Can you work these out from the model? Positions are in its coordinate system, mm. Face numbers are marked on the shaded views. Round coordinates to 2 decimals unless told otherwise and drop trailing zeros. Loops run counter-clockwise (first coordinate to the right, second up) from the corner with the lowest first, then second, coordinate; pieces in that order, holes last. Notation, with made-up numbers: M 34,22 L 59,22 A25 ccw 59,54 Z; hole C -14.5,61 d1. An arc over 180 degrees is marked long. Return JSON: item names as keys, results as strings.
```python
from build123d import *

# Parameters (mm, degrees)
ESQUISSE1_R                = 20
ESQUISSE1_R_2              = 12
ESQUISSE1_R_3              = 1.15
BOSS_EXTRU_1_DEPTH         = 4
PER_AGEAVANC_1_OUTLINE_R   = 2.2
PER_AGEAVANC_1_OUTLINE_R_2 = 1.15
PER_AGEAVANC_1_DEPTH       = 2
BOSS_EXTRU_2_START         = -4
ESQUISSE3_R                = 13.45
ESQUISSE3_R_2              = 12
BOSS_EXTRU_2_DEPTH         = 2.3
CHANFREIN1_SIZE            = 0.5
CHANFREIN2_SIZE            = 1


# Read off the part's stored shape, not the designer's step: PerçageAvancé1
with BuildPart() as part:
    # Esquisse1 → Boss.-Extru.1 (new body)
    with BuildSketch(Plane(origin=(0, 0, 0), x_dir=(1, 0, 0), z_dir=(0, 1, 0))):
        with Locations(Location((0, 0, 0), (0, 0, 270))):
            Circle(ESQUISSE1_R)
        with Locations(Location((0, 0, 0), (0, 0, 270))):
            Circle(ESQUISSE1_R_2, mode=Mode.SUBTRACT)
        with Locations(Location((-14.289419162, -8.25, 0), (0, 0, 270))):
            Circle(ESQUISSE1_R_3, mode=Mode.SUBTRACT)
        with Locations(Location((14.289419162, -8.25, 0), (0, 0, 270))):
            Circle(ESQUISSE1_R_3, mode=Mode.SUBTRACT)
        with Locations(Location((0, 16.5, 0), (0, 0, 270))):
            Circle(ESQUISSE1_R_3, mode=Mode.SUBTRACT)
    extrude(amount=BOSS_EXTRU_1_DEPTH)

    # PerçageAvancé1 outline → PerçageAvancé1 (cut)
    # profile 1 of 3: a face of its own
    with BuildSketch(Plane(origin=(0, 0, 0), x_dir=(1, 0, 0), z_dir=(0, 1, 0))):
        with Locations((-14.289419162, -8.25)):
            Circle(PER_AGEAVANC_1_OUTLINE_R)
        with Locations((-14.289419162, -8.25)):
            Circle(PER_AGEAVANC_1_OUTLINE_R_2, mode=Mode.SUBTRACT)
    # profile 2 of 3: a face of its own
    with BuildSketch(Plane(origin=(0, 0, 0), x_dir=(1, 0, 0), z_dir=(0, 1, 0))):
        with Locations((14.289419162, -8.25)):
            Circle(PER_AGEAVANC_1_OUTLINE_R)
        with Locations((14.289419162, -8.25)):
            Circle(PER_AGEAVANC_1_OUTLINE_R_2, mode=Mode.SUBTRACT)
    # profile 3 of 3: a face of its own
    with BuildSketch(Plane(origin=(0, 0, 0), x_dir=(1, 0, 0), z_dir=(0, 1, 0))):
        with Locations((0, 16.5)):
            Circle(PER_AGEAVANC_1_OUTLINE_R)
        with Locations((0, 16.5)):
            Circle(PER_AGEAVANC_1_OUTLINE_R_2, mode=Mode.SUBTRACT)
    extrude(amount=PER_AGEAVANC_1_DEPTH, mode=Mode.SUBTRACT)

    # Esquisse3 → Boss.-Extru.2 (add)
    with BuildSketch(Plane.XZ.offset(BOSS_EXTRU_2_START)):
        with Locations(Location((0, 0, 0), (0, 0, 90))):
            Circle(ESQUISSE3_R)
        with Locations(Location((0, 0, 0), (0, 0, 90))):
            Circle(ESQUISSE3_R_2, mode=Mode.SUBTRACT)
    extrude(amount=-BOSS_EXTRU_2_DEPTH)

    # Chanfrein1
    chanfrein1_edges = [part.edges().sort_by_distance(p)[0] for p in [
        (0, 6.3, -12),
    ]]
    chamfer(chanfrein1_edges, length=CHANFREIN1_SIZE)

    # Chanfrein2
    chanfrein2_edges = [part.edges().sort_by_distance(p)[0] for p in [
        (0, 4, -20),
        (0, 0, -20),
        (0, 0, -12),
    ]]
    chamfer(chanfrein2_edges, length=CHANFREIN2_SIZE)


solid = part.part
```
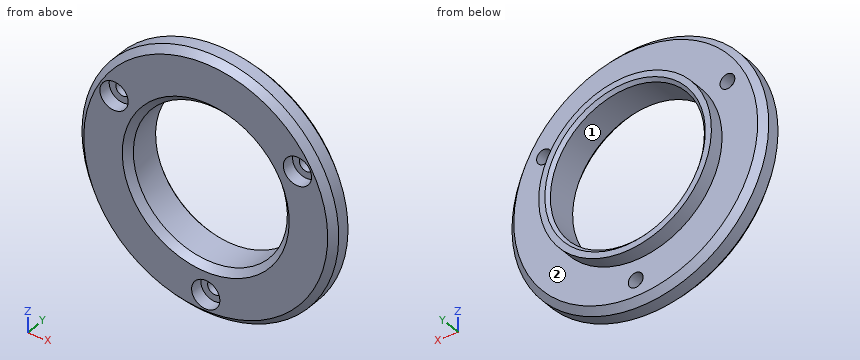
Q1. Suppose I cut it at C-C, the plane y = 1.5. Please give me the cut outline in (x, z), plus the area to 3 significant figures.
Results:
{"outline": "C 0,0 d40; hole C -14.29,8.25 d4.4; hole C 0,0 d24; hole C 0,-16.5 d4.4; hole C 14.29,8.25 d4.4", "area": "759 mm2"}
Q2. Suppose I cut it at B-B, the plane x = 0. Please give me the cut outline in (y, z).
Results:
{"outline": "M 0,-19 L 1,-20 L 3,-20 L 4,-19 L 4,-17.65 L 2,-17.65 L 2,-18.7 L 0,-18.7 Z; M 0,-14.3 L 2,-14.3 L 2,-15.35 L 4,-15.35 L 4,-13.45 L 6.3,-13.45 L 6.3,-12.5 L 5.8,-12 L 1,-12 L 0,-13 Z; M 0,13 L 1,12 L 5.8,12 L 6.3,12.5 L 6.3,13.45 L 4,13.45 L 4,19 L 3,20 L 1,20 L 0,19 Z"}
Q3. Suppose I cut it at D-D, the plane y = 4.5. Please give me the cut outline in (x, z).
Results:
{"outline": "C 0,0 d26.9; hole C 0,0 d24"}
Q4. I'm going to push flat-ended pins straight in: pin 1 Ø1.3 at (x, z) = (13.5, 7.5) entering from -Y; pin 2 Ø1.4 at (x, z) = (-14.29, 8.25) entering from +Y; pin 3 Ø4 at (x, z) = (-15, 8.5) entering from +Y; pin 4 Ø2 at (y, z) = (1, 2.5) entering from -X. Where does each tip first touch, or does it pass through?
Results:
{"pin 1": "stops at y = 2", "pin 2": "passes through", "pin 3": "stops at y = 4", "pin 4": "stops at x = -19.94"}
Q5. Thinking about a two-plate mould opening in Z: for the marked faces 1 and 2, which applies, pulls with the +Z half, pulls with the -Z half, needs draft (parallel to the pull), parting line crosses it, or undercut?
Results:
{"face 1": "undercut", "face 2": "needs draft"}
Q6. If I drill on line 1 along X through (y, z) = (3.15, 8.25); line 2 along X through (y, z) = (2.5, 8.25); line 3 along Y through (x, z) = (7, 14), over which ranges is the centre line in solid material (lowest first)?
Results:
{"line 1": "x = -18.05 to -15.44, -13.14 to -8.71, 8.71 to 13.14, 15.44 to 18.05", "line 2": "x = -18.22 to -15.44, -13.14 to -8.71, 8.71 to 13.14, 15.44 to 18.22", "line 3": "y = 0 to 4"}
Q7. Suppose I cut it at A-A, the plane z = 0. Please give me the cut outline in (x, y), plus the area to 3 significant figures.
Results:
{"outline": "M -20,1 L -19,0 L -13,0 L -12,1 L -12,5.8 L -12.5,6.3 L -13.45,6.3 L -13.45,4 L -19,4 L -20,3 Z; M 12,1 L 13,0 L 19,0 L 20,1 L 20,3 L 19,4 L 13.45,4 L 13.45,6.3 L 12.5,6.3 L 12,5.8 Z", "area": "67.4 mm2"}
